Geometry check sheet. Reference: drawing and pictorial views, mm from the part's lowest x, y, z. A direction names the side the tool comes from. Give positions to 0.01 mm unless a question says otherwise; leave off trailing zeros. Order: outer loops, then holes, each group sorted by start corner. A loop starts at its lowest first (then second) coordinate and runs counter-clockwise, first axis right, second up.
Item 1: Sectioned sample at C-C on z = 4.2. Record the boundary of the cut face in (x, y), and give its area (3 significant figures).
Item 2: Sectioned sample at A-A on x = 62. Record the boundary of the cut face in (y, z).
Item 3: Access from +Z, -Z, +X, -X, +Y, -Y to the whole of each face (thin tool, end or side, straight path). Record for the marked faces 1, 2 and 3.
Item 4: Sectioned sample at D-D on x = 38. Record the boundary of the cut face in (y, z).
Item 5: Material ranges on line 1 along X through (y, z) = (1.15, 12); line 2 along Z through (x, y) = (38, 14.5); line 3 along Z through (x, y) = (28.5, 14.75), recorded low to high.
Item 6: Sectioned sample at B-B on y = 5.75. Record the boundary of the cut face in (x, z) (3 decimals).
Item 7: Gauge pin test, flat ends, axial feed: P1, Ø5, axis at x = 70.5, z = 7.5, coming from the +Y side; P2, Ø3.5, axis at y = 9, z = 8, coming from the +X side; P3, Ø8, axis at x = 26, z = 8.5, coming from the -Y side; P4, Ø2.5, axis at x = 47.5, z = 12, coming from the -Y side. Record the tip position at first contact, or that the pin passes through.
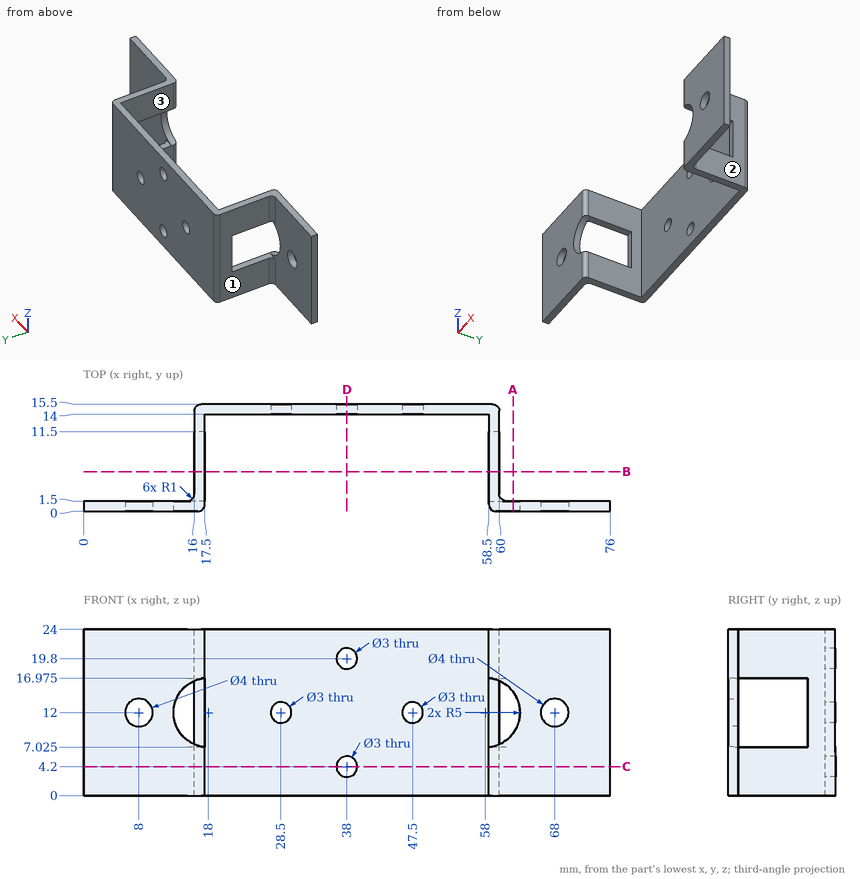
Report:
1. outline: (0, 0) - (16.5, 0) arc R1 ccw to (17.5, 1) - (17.5, 14) - (36.5, 14) - (36.5, 15.5) - (17, 15.5) arc R1 ccw to (16, 14.5) - (16, 2.5) arc R1 cw to (15, 1.5) - (0, 1.5) - close; (39.5, 14) - (58.5, 14) - (58.5, 1) arc R1 ccw to (59.5, 0) - (76, 0) - (76, 1.5) - (61, 1.5) arc R1 cw to (60, 2.5) - (60, 14.5) arc R1 ccw to (59, 15.5) - (39.5, 15.5) - close
1. area: 151 mm2
2. outline: (0, 0) - (1.5, 0) - (1.5, 9) - (0, 9) - close; (0, 15) - (1.5, 15) - (1.5, 24) - (0, 24) - close
3. face 1: +Z, -Z, -X, +Y
3. face 2: +Z, -Z, +X, +Y
3. face 3: +Z, -Z, -Y
4. outline: (14, 0) - (15.5, 0) - (15.5, 2.7) - (14, 2.7) - close; (14, 5.7) - (15.5, 5.7) - (15.5, 18.3) - (14, 18.3) - close; (14, 21.3) - (15.5, 21.3) - (15.5, 24) - (14, 24) - close
5. line 1: x = 0 to 6, 10 to 13, 63 to 66, 70 to 76
5. line 2: z = 0 to 2.7, 5.7 to 18.3, 21.3 to 24
5. line 3: z = 0 to 10.5, 13.5 to 24
6. outline: (16, 0) - (17.5, 0) - (17.5, 7.025) - (16, 7.025) - close; (16, 16.975) - (17.5, 16.975) - (17.5, 24) - (16, 24) - close; (58.5, 0) - (60, 0) - (60, 7.025) - (58.5, 7.025) - close; (58.5, 16.975) - (60, 16.975) - (60, 24) - (58.5, 24) - close
7. P1: stops at y = 1.5
7. P2: stops at x = 60
7. P3: stops at y = 14
7. P4: passes through
